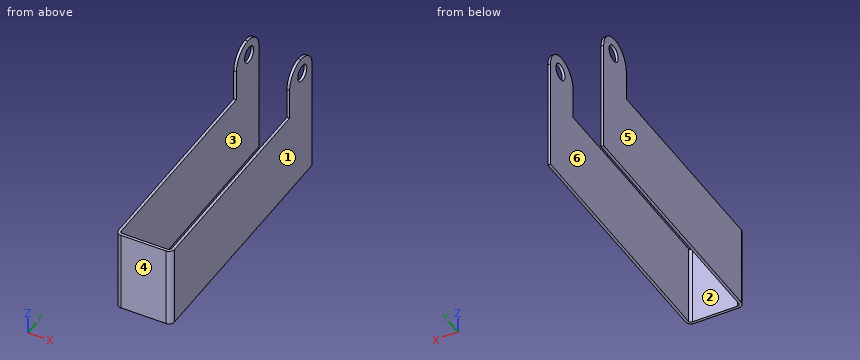
```python
from build123d import *

# Parameters (mm, degrees)
SKETCH1_W                      = 18.53
SKETCH1_H                      = 1
BASE_FLANGE1_DEPTH             = 30
EDGE_FLANGE1_STRIP_W           = 6
EDGE_FLANGE1_STRIP_H           = 1
EDGE_FLANGE1_STRIP_CUT_DEPTH   = 30
EDGE_FLANGE1_STRIP_2_W         = 6
EDGE_FLANGE1_STRIP_2_H         = 1
EDGE_FLANGE1_STRIP_CUT_2_DEPTH = 30
EDGE_FLANGE1_DEPTH             = 30
EDGE_FLANGE1_BEND_DEPTH        = 30
SKETCH17_W                     = 18.97
SKETCH17_H                     = 15
TAB1_DEPTH                     = 1
SKETCH24_R                     = 3
CUT_EXTRUDE1_DEPTH             = 107.692049376
FILLET1_R                      = 7.5


# Sheet-metal steps are written as plain solids
with BuildPart() as part:
    # Sketch1 → Base-Flange1 (new body)
    with BuildSketch(Plane.XY):
        with Locations((9.265, -0.5)):
            Rectangle(SKETCH1_W, SKETCH1_H)
    extrude(amount=BASE_FLANGE1_DEPTH)

    # Edge-Flange1 strip (across the edge) → Edge-Flange1 strip cut (cut)
    with BuildSketch(Plane(origin=(18.53, 0, 30), x_dir=(-1, 0, 0), z_dir=(0, 0, -1))):
        with Locations((-2, -0.5)):
            Rectangle(EDGE_FLANGE1_STRIP_W, EDGE_FLANGE1_STRIP_H)
    extrude(amount=EDGE_FLANGE1_STRIP_CUT_DEPTH, mode=Mode.SUBTRACT)

    # Edge-Flange1 strip 2 (across the edge) → Edge-Flange1 strip cut 2 (cut)
    with BuildSketch(Plane.XY):
        with Locations((-2, -0.5)):
            Rectangle(EDGE_FLANGE1_STRIP_2_W, EDGE_FLANGE1_STRIP_2_H)
    extrude(amount=EDGE_FLANGE1_STRIP_CUT_2_DEPTH, mode=Mode.SUBTRACT)

    # Edge-Flange1 section (across the edge) → Edge-Flange1 (add)
    with BuildSketch(Plane(origin=(18.53, 0, 30), x_dir=(-1, 0, 0), z_dir=(0, 0, -1))):
        with BuildLine():
            Line((-1, 1), (-1, 92.54))
            Line((-1, 92.54), (0, 92.54))
            Line((0, 92.54), (0, 1))
            ThreePointArc((0, 1), (0.292893219, 0.292893219), (1, 0))
            Line((1, 0), (1, -1))
            ThreePointArc((1, -1), (-0.414213562, -0.414213562), (-1, 1))
        make_face()
    extrude(amount=EDGE_FLANGE1_DEPTH)

    # Edge-Flange1 section 2 (across the edge) → Edge-Flange1 bend (add)
    with BuildSketch(Plane.XY):
        with BuildLine():
            Line((-1, 1), (-1, 92.54))
            Line((-1, 92.54), (0, 92.54))
            Line((0, 92.54), (0, 1))
            ThreePointArc((0, 1), (0.292893219, 0.292893219), (1, 0))
            Line((1, 0), (1, -1))
            ThreePointArc((1, -1), (-0.414213562, -0.414213562), (-1, 1))
        make_face()
    extrude(amount=EDGE_FLANGE1_BEND_DEPTH)

    # Sketch17 → Tab1 (add)
    with BuildSketch(Plane(origin=(19.53, 0, 0), x_dir=(0, 0, -1), z_dir=(1, 0, 0))):
        with Locations((-39.485, 85.04)):
            Rectangle(SKETCH17_W, SKETCH17_H)
    tab1 = extrude(amount=-TAB1_DEPTH)

    # Mirror1: Tab1 across plane
    add(tab1.mirror(Plane(origin=(9.265, 0, 0), x_dir=(0, 0, 1), z_dir=(1, 0, 0))))

    # Sketch24 → Cut-Extrude1 (cut, through all)
    with BuildSketch(Plane(origin=(19.53, 0, 0), x_dir=(0, 0, -1), z_dir=(1, 0, 0))):
        with Locations(Location((-42.746376896, 85.96, 0), (0, 0, 90))):
            Circle(SKETCH24_R)
    extrude(amount=-CUT_EXTRUDE1_DEPTH, mode=Mode.SUBTRACT)

    # Fillet1
    fillet1_edges = [part.edges().sort_by_distance(p)[0] for p in [
        (19.03, 77.54, 48.97),
        (-0.5, 77.54, 48.97),
        (-0.5, 92.54, 48.97),
        (19.03, 92.54, 48.97),
    ]]
    fillet(fillet1_edges, radius=FILLET1_R - 0.0001)  # a hair under: the kernel refuses the full size


solid = part.part
```
Part model, mm, in its own coordinate system. Face numbers are marked on the shaded views. A direction names the side the tool comes from. Give positions to 0.01 mm unless a question says otherwise; leave off trailing zeros. Order: outer loops, then holes, each group sorted by start corner. A loop starts at its lowest first (then second) coordinate and runs counter-clockwise, first axis right, second up. Notation, with made-up numbers: M 12.5,-21 L 21.5,-21 A32 ccw 21.5,15 Z; hole C -17.75,79.25 d4. An arc over 180 degrees is marked long. Use a Markdown table: item, result. Add a question column.
(1) Saw through at D-D, the plane x = 12.25. Give the cut face in (y, z).
(2) Saw through at A-A, the plane z = 33. Give the cut face in (x, y), and give its area (3 significant figures).
(3) Saw through at C-C, the plane y = 85.96. Give the cut face in (x, z).
(4) Mould opens along X. For the marked faces 1, 2, 3 and 4 say: +X half, -X half, draft (parallel to the pull), parting line (faces both ways), or undercut.
(5) Drop flat-ended pins along their axis: P1, Ø6, axis at x = 17.5, z = 30.5, coming from the +Y side; P2, Ø8.5, axis at x = 9, z = 12.5, coming from the +Y side; P3, Ø0.5, axis at x = -0.5, z = 33.5, coming from the -Y side. Give the stop position or say it passes through.
(6) Saw through at B-B, the plane y = 48.5. Give the cut face in (x, z).
(7) Probe line 1 along X through (y, z) = (76.5, 4); line 2 along Y through (x, z) = (15, 28.5); line 3 along Z through (x, y) = (-0.3, 85.96). List the from-to ranges inside material, lowest first. Write a range as [from, to].
(8) 3-axis set-ups, long thin cutter, end or side, ignore diameter. For the marked faces 5 and 6: which of +Z, -Z, +X, -X, +Y, -Y reach the whole face in a straight line?
Answer key:
| question | item | result |
|---|---|---|
| 1 | outline | M -1,0 L 0,0 L 0,30 L -1,30 Z |
| 2 | outline | M -1,77.54 L 0,77.54 L 0,92.54 L -1,92.54 Z; M 18.53,77.54 L 19.53,77.54 L 19.53,92.54 L 18.53,92.54 Z |
| 2 | area | 30.0 mm^2 |
| 3 | outline | M -1,0 L 0,0 L 0,39.75 L -1,39.75 Z; M -1,45.75 L 0,45.75 L 0,48.91 L -1,48.91 Z; M 18.53,0 L 19.53,0 L 19.53,39.75 L 18.53,39.75 Z; M 18.53,45.75 L 19.53,45.75 L 19.53,48.91 L 18.53,48.91 Z |
| 4 | face 1 | +X half |
| 4 | face 2 | undercut |
| 4 | face 3 | undercut |
| 4 | face 4 | draft |
| 5 | P1 | y = 92.54 |
| 5 | P2 | y = 0 |
| 5 | P3 | y = 77.54 |
| 6 | outline | M -1,0 L 0,0 L 0,30 L -1,30 Z; M 18.53,0 L 19.53,0 L 19.53,30 L 18.53,30 Z |
| 7 | line 1 | [-1, 0], [18.53, 19.53] |
| 7 | line 2 | [-1, 0] |
| 7 | line 3 | [0, 39.75], [45.75, 48.91] |
| 8 | face 5 | +Z, -Z, -X, +Y, -Y |
| 8 | face 6 | +Z, -Z, +Y |
